CAD build for the part. Positions are in the model's coordinates, mm. A direction names the side the tool comes from. Coordinates: 2 decimals unless noted, no trailing zeros. Write each loop counter-clockwise with the first axis right and the second up, starting at its lowest first coordinate (ties: lowest second). Pieces come first, ordered by that corner, then holes. Notation, with made-up numbers: (19.5, 70.25) -> (77.5, 70.25) arc R17 cw to (77.5, 80.25) -> close; hole circle Ø9 at (18.5, -3.75). An arc over 180 degrees is marked (long way). Answer as CSV lines item,"result".
```python
from build123d import *

# Parameters (mm, degrees)
SKETCH1_W           = 177.8
SKETCH1_H           = 114.3
BOSS_EXTRUDE1_DEPTH = 25.4
SKETCH3_R           = 3.3782
CUT_EXTRUDE2_DEPTH  = 109.694491581
SKETCH4_W           = 157.48
SKETCH4_H           = 81.28
CUT_EXTRUDE3_DEPTH  = 12.7
SKETCH3_3_R         = 6.35
SKETCH3_3_R_2       = 3.3782
CUT_EXTRUDE4_DEPTH  = 12.7
FILLET4_R           = 20.32
FILLET7_R           = 15.24
FILLET8_R           = 7.62


with BuildPart() as part:
    # Sketch1 → Boss-Extrude1 (new body)
    with BuildSketch(Plane(origin=(0, 0, 0), x_dir=(1, 0, 0), z_dir=(0, 1, 0))):
        Rectangle(SKETCH1_W, SKETCH1_H)
    extrude(amount=BOSS_EXTRUDE1_DEPTH)

    # Sketch3 → Cut-Extrude2 (cut, through all)
    with BuildSketch(Plane(origin=(0, 25.4, 0), x_dir=(1, 0, 0), z_dir=(0, 1, 0))):
        with Locations(Location((76.2, -40.64, 0), (0, 0, 270))):
            Circle(SKETCH3_R)
        with Locations(Location((76.2, 40.64, 0), (0, 0, 270))):
            Circle(SKETCH3_R)
        with Locations(Location((-76.2, -40.64, 0), (0, 0, 270))):
            Circle(SKETCH3_R)
        with Locations(Location((-76.2, 40.64, 0), (0, 0, 270))):
            Circle(SKETCH3_R)
    extrude(amount=-CUT_EXTRUDE2_DEPTH, mode=Mode.SUBTRACT)

    # Sketch4 → Cut-Extrude3 (cut)
    with BuildSketch(Plane(origin=(0, 25.4, 0), x_dir=(1, 0, 0), z_dir=(0, 1, 0))):
        Rectangle(SKETCH4_W, SKETCH4_H)
    extrude(amount=-CUT_EXTRUDE3_DEPTH, mode=Mode.SUBTRACT)

    # Sketch3<3> → Cut-Extrude4 (cut)
    # profile 1 of 4: a face of its own
    with BuildSketch(Plane(origin=(0, 25.4, 0), x_dir=(1, 0, 0), z_dir=(0, 1, 0))):
        with Locations((76.2, 40.64)):
            Circle(SKETCH3_3_R)
        with Locations(Location((76.2, 40.64, 0), (0, 0, 270))):
            Circle(SKETCH3_3_R_2, mode=Mode.SUBTRACT)
    # profile 2 of 4: a face of its own
    with BuildSketch(Plane(origin=(0, 25.4, 0), x_dir=(1, 0, 0), z_dir=(0, 1, 0))):
        with Locations((76.2, -40.64)):
            Circle(SKETCH3_3_R)
        with Locations(Location((76.2, -40.64, 0), (0, 0, 270))):
            Circle(SKETCH3_3_R_2, mode=Mode.SUBTRACT)
    # profile 3 of 4: a face of its own
    with BuildSketch(Plane(origin=(0, 25.4, 0), x_dir=(1, 0, 0), z_dir=(0, 1, 0))):
        with Locations((-76.2, -40.64)):
            Circle(SKETCH3_3_R)
        with Locations(Location((-76.2, -40.64, 0), (0, 0, 270))):
            Circle(SKETCH3_3_R_2, mode=Mode.SUBTRACT)
    # profile 4 of 4: a face of its own
    with BuildSketch(Plane(origin=(0, 25.4, 0), x_dir=(1, 0, 0), z_dir=(0, 1, 0))):
        with Locations((-76.2, 40.64)):
            Circle(SKETCH3_3_R)
        with Locations(Location((-76.2, 40.64, 0), (0, 0, 270))):
            Circle(SKETCH3_3_R_2, mode=Mode.SUBTRACT)
    extrude(amount=-CUT_EXTRUDE4_DEPTH, mode=Mode.SUBTRACT)

    # Fillet4
    # the kernel refuses this fillet: 20.32 mm, written as the material it takes off along each edge
    with BuildSketch(Plane(origin=(88.9, 25.4, 107.95), x_dir=(-1, 0, 0), z_dir=(0, 0, -1)), Plane(origin=(-88.9, 25.4, -107.95), x_dir=(1, 0, 0), z_dir=(0, 0, 1))) as fillet4_piece_1:
        with BuildLine():
            CenterArc((FILLET4_R, -FILLET4_R), FILLET4_R, 90, 90)
            Line((0, -FILLET4_R), (0, 0))
            Line((0, 0), (FILLET4_R, 0))
        make_face()
    extrude(amount=215.9, mode=Mode.SUBTRACT)

    # Fillet7
    # the kernel refuses this fillet: 15.24 mm, written as the material it takes off along each edge
    with BuildSketch(Plane(origin=(-68.58, 25.4, 57.15), x_dir=(0, -1, 0), z_dir=(1, 0, 0))) as fillet7_piece_1:
        with BuildLine():
            CenterArc((FILLET7_R, FILLET7_R), FILLET7_R, 180, 90)
            Line((0, FILLET7_R), (0, 0))
            Line((0, 0), (FILLET7_R, 0))
        make_face()
    extrude(amount=137.16, mode=Mode.SUBTRACT)
    with BuildSketch(Plane(origin=(88.9, -38.1, 57.15), x_dir=(-1, 0, 0), z_dir=(0, 1, 0))) as fillet7_piece_2:
        with BuildLine():
            CenterArc((FILLET7_R, -FILLET7_R), FILLET7_R, 90, 90)
            Line((0, -FILLET7_R), (0, 0))
            Line((0, 0), (FILLET7_R, 0))
        make_face()
    extrude(amount=43.18, mode=Mode.SUBTRACT)
    with BuildSketch(Plane(origin=(-88.9, -38.1, 57.15), x_dir=(1, 0, 0), z_dir=(0, 1, 0))) as fillet7_piece_3:
        with BuildLine():
            CenterArc((FILLET7_R, FILLET7_R), FILLET7_R, 180, 90)
            Line((0, FILLET7_R), (0, 0))
            Line((0, 0), (FILLET7_R, 0))
        make_face()
    extrude(amount=43.18, mode=Mode.SUBTRACT)
    with BuildSketch(Plane(origin=(-68.58, 5.08, 57.15), x_dir=(-1, 0, 0), z_dir=(0, -1, 0))) as fillet7_piece_4:
        with BuildLine():
            CenterArc((20.32 - FILLET7_R, FILLET7_R), FILLET7_R, 270, 90)
            Line((20.32, FILLET7_R), (20.32, 0))
            Line((20.32, 0), (20.32 - FILLET7_R, 0))
        make_face()
    revolve(axis=Axis((-68.58, 5.08, 57.15), (0, 0, -1)), revolution_arc=90, mode=Mode.SUBTRACT)
    with BuildSketch(Plane(origin=(68.58, 5.08, 57.15), x_dir=(1, 0, 0), z_dir=(0, -1, 0))) as fillet7_piece_5:
        with BuildLine():
            CenterArc((20.32 - FILLET7_R, -FILLET7_R), FILLET7_R, 0, 90)
            Line((20.32, -FILLET7_R), (20.32, 0))
            Line((20.32, 0), (20.32 - FILLET7_R, 0))
        make_face()
    revolve(axis=Axis((68.58, 5.08, 57.15), (0, 0, 1)), revolution_arc=90, mode=Mode.SUBTRACT)

    # Fillet8
    fillet8_edges = [part.edges().sort_by_distance(p)[0] for p in [
        (0, 25.4, -57.15),
        (-88.9, 2.54, -57.15),
        (88.9, 2.54, -57.15),
        (-82.948409794, 19.448409794, -57.15),
        (82.948409794, 19.448409794, -57.15),
    ]]
    fillet(fillet8_edges, radius=FILLET8_R)


solid = part.part
```
Item 1: Saw through at B-B on z = 9. Give the cut face in (x, y), and give its area (3 significant figures).
Answer below:
outline,"(-88.9, 0) -> (88.9, 0) -> (88.9, 5.08) arc R20.32 ccw to (78.74, 22.68) -> (78.74, 12.7) -> (-78.74, 12.7) -> (-78.74, 22.68) arc R20.32 ccw to (-88.9, 5.08) -> close"
area,"2,360 mm2"
Item 2: Saw through at A-A on x = -32.5. Give the cut face in (y, z), and give its area (3 significant figures).
Answer below:
outline,"(0, -57.15) -> (17.78, -57.15) arc R7.62 ccw to (25.4, -49.53) -> (25.4, -40.64) -> (12.7, -40.64) -> (12.7, 40.64) -> (25.4, 40.64) -> (25.4, 41.91) arc R15.24 ccw to (10.16, 57.15) -> (0, 57.15) -> close"
area,"1,810 mm2"
Item 3: Two-plate mould, pull along X, no slides. Class faces 3 (the flat face through (-88.9, 3, -3)), 4 (the flat face through (-1, 19, 40.64)), 5 (the flat face through (88.9, 3, -3)): pulls with the +X half, pulls with the -X half, needs draft (parallel to the pull), parting line crosses it, or undercut.
Answer below:
face 3,"pulls with the -X half"
face 4,"undercut"
face 5,"pulls with the +X half"
Item 4: 3-axis set-ups, long thin cutter, end or side, ignore diameter. For faces 1 (the flat face through (-1, 0, -1)), 2 (the cylindrical face through (77.035, 17.712, -46.935)): which of +Z, -Z, +X, -X, +Y, -Y reach the whole face in a straight line?
Answer below:
face 1,"+Z, -Z, +X, -X, -Y"
face 2,"+Y"
Item 5: Flat gauge pins, fed straight in: pin 1 (6 mm diameter, centred on x = 13.5, z = -10, fed in from +Y); pin 2 (3 mm diameter, centred on y = 13, z = 28.5, fed in from -X); pin 3 (6 mm diameter, centred on x = -14, z = -9, fed in from -Y); pin 4 (6 mm diameter, centred on x = 76.2, z = -40.64, fed in from +Y). Where does each tip first touch, or does it go through?
Answer below:
pin 1,"stops at y = 12.7"
pin 2,"stops at x = -87.86"
pin 3,"stops at y = 0"
pin 4,"passes through"
Item 6: Saw through at C-C on x = 76.2. State how many separate pieces and enclosed holes the cut face has, and give its area (3 significant figures).
Answer below:
separate pieces,"3"
enclosed holes,"0"
area,"1,440 mm2"
Item 7: Wall check: line 1 (X direction, y = 9.25, z = -40.64); line 2 (Z direction, x = 77, y = 5.75); line 3 (X direction, y = 10, z = 40.64). Give the ranges that are in metal, low to high. Write a range as from..to.
Answer below:
line 1,"x = -88.47..-79.58, -72.82..72.82, 79.58..88.47"
line 2,"z = -57.15..-43.92, -37.36..37.36, 43.92..56.77"
line 3,"x = -88.3..-79.58, -72.82..72.82, 79.58..88.3"
